Can you work these out from the drawing? Everything is in mm from the part's minimum corner. Coordinates: 2 decimals unless noted, no trailing zeros. Order: outer loops, then holes, each group sorted by start corner. A loop starts at its lowest first (then second) coordinate and runs counter-clockwise, first axis right, second up. Notation, with made-up numbers: (0, 23) -> (43, 23) arc R20 cw to (43, 57) -> close; hole circle Ø3 at (50.5, 6). An arc over 180 degrees is marked (long way). Return JSON: item names as keys, results as strings. Group by question number.
1) If we section it at D-D, the plane z = 0.6: Please give me the cut outline in (x, y), then the cut area to 3 significant figures.
2) If I drill on probe 1 along X at (y, z) = (5.25, 0.7); probe 2 along Y at (x, z) = (25, 0.4); probe 3 along X at (y, z) = (12, 0.75), over which ranges is the centre line in solid material (lowest first)? Write a range as from..to.
3) If we section it at A-A, the plane y = 12: Please give me the cut outline in (x, z), then the cut area to 3 significant figures.
4) If we section it at B-B, the plane x = 46: Please give me the cut outline in (y, z).
5) If we section it at C-C, the plane y = 5.25: Please give me the cut outline in (x, z).
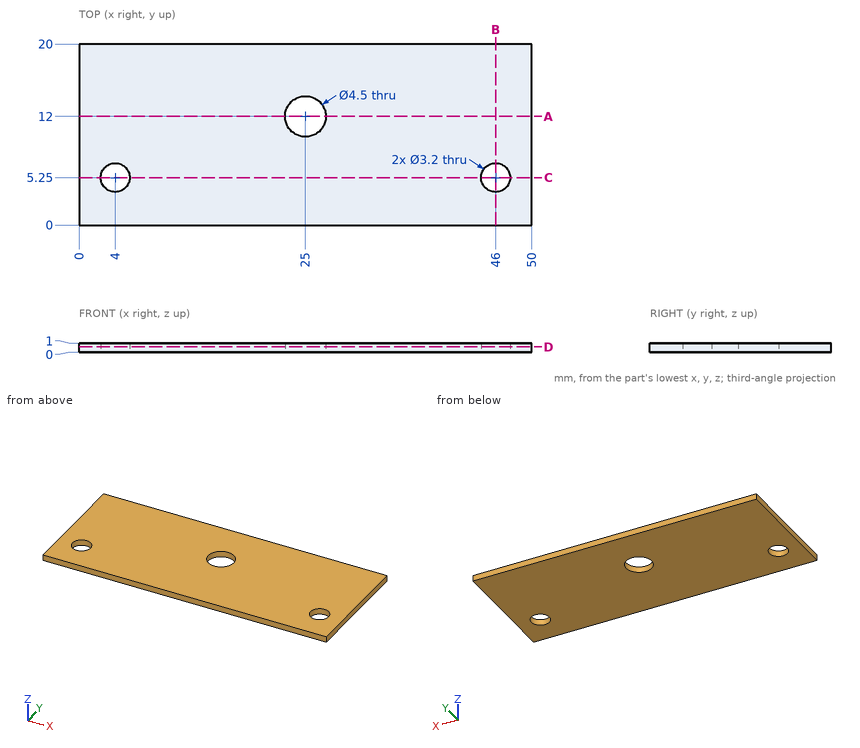
Result sheet:
{
 "1": {"outline": "(0, 0) -> (50, 0) -> (50, 20) -> (0, 20) -> close; hole circle Ø3.2 at (4, 5.25); hole circle Ø4.5 at (25, 12); hole circle Ø3.2 at (46, 5.25)", "area": "968 mm2"},
 "2": {"probe 1": "x = 0..2.4, 5.6..44.4, 47.6..50", "probe 2": "y = 0..9.75, 14.25..20", "probe 3": "x = 0..22.75, 27.25..50"},
 "3": {"outline": "(0, 0) -> (22.75, 0) -> (22.75, 1) -> (0, 1) -> close; (27.25, 0) -> (50, 0) -> (50, 1) -> (27.25, 1) -> close", "area": "45.5 mm2"},
 "4": {"outline": "(0, 0) -> (3.65, 0) -> (3.65, 1) -> (0, 1) -> close; (6.85, 0) -> (20, 0) -> (20, 1) -> (6.85, 1) -> close"},
 "5": {"outline": "(0, 0) -> (2.4, 0) -> (2.4, 1) -> (0, 1) -> close; (5.6, 0) -> (44.4, 0) -> (44.4, 1) -> (5.6, 1) -> close; (47.6, 0) -> (50, 0) -> (50, 1) -> (47.6, 1) -> close"}
}
